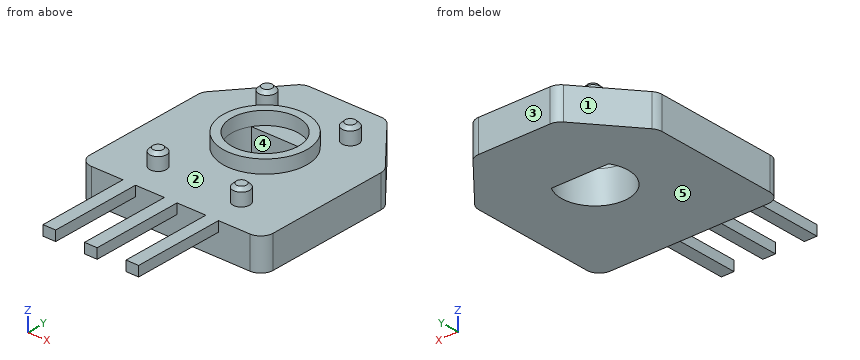
```python
from build123d import *
from build123d.topology import SkipClean

# Parameters (mm, degrees)
BOSS_EXTRUDE1_DEPTH = 1.93
SKETCH2_R           = 2.5
SKETCH2_R_2         = 2
BOSS_EXTRUDE2_DEPTH = 0.79
FILLET2_R           = 0.75
SKETCH5_R           = 0.5
BOSS_EXTRUDE4_DEPTH = 0.97
CHAMFER1_SIZE       = 0.2
SKETCH6_W           = 0.76
SKETCH6_H           = 0.6
BOSS_EXTRUDE5_DEPTH = 5.5


with BuildPart() as part:
    # Sketch1 → Boss-Extrude1 (new body)
    with BuildSketch(Plane.XY):
        Polygon((5.5, 0), (5.5, -6.5), (-5.5, -6.5), (-5.5, 0), (-5.5, 1.96), (-2.49602332, 5.54), (2.49602332, 5.54), (5.5, 1.96), align=None)
        with BuildLine():
            Line((-1.718566554, 1.023), (1.718566554, 1.023))
            ThreePointArc((1.718566554, 1.023), (0, -2), (-1.718566554, 1.023))
        make_face(mode=Mode.SUBTRACT)
    extrude(amount=BOSS_EXTRUDE1_DEPTH)

    # Sketch2 → Boss-Extrude2 (add)
    with SkipClean():  # the faces are left unmerged after this step: merging them gives an invalid solid
        with BuildSketch(Plane.XY.offset(1.93)):
            with Locations(Location((0, 0, 0), (0, 0, 180))):
                Circle(SKETCH2_R)
            with Locations(Location((0, 0, 0), (0, 0, 149.236204264))):
                Circle(SKETCH2_R_2, mode=Mode.SUBTRACT)
        extrude(amount=BOSS_EXTRUDE2_DEPTH)

    # Fillet2
    fillet2_edges = [part.edges().sort_by_distance(p)[0] for p in [
        (5.5, -6.5, 0.965),
        (-5.5, -6.5, 0.965),
        (-5.5, 1.96, 0.965),
        (-2.49602332, 5.54, 0.965),
        (2.49602332, 5.54, 0.965),
        (5.5, 1.96, 0.965),
    ]]
    fillet(fillet2_edges, radius=FILLET2_R)

    # Sketch5 → Boss-Extrude4 (add)
    with SkipClean():  # the faces are left unmerged after this step: merging them gives an invalid solid
        with BuildSketch(Plane.XY.offset(1.93)):
            with Locations(Location((-2.5, -4.5, 0), (0, 0, 180))):
                Circle(SKETCH5_R)
            with Locations(Location((2.5, -4.5, 0), (0, 0, 180))):
                Circle(SKETCH5_R)
            with Locations(Location((2.5, 3, 0), (0, 0, 180))):
                Circle(SKETCH5_R)
            with Locations(Location((-2.5, 3, 0), (0, 0, 180))):
                Circle(SKETCH5_R)
        extrude(amount=BOSS_EXTRUDE4_DEPTH)

    # Chamfer1
    chamfer1_edges = [part.edges().sort_by_distance(p)[0] for p in [
        (3, -4.5, 2.9),
        (-2, -4.5, 2.9),
        (3, 3, 2.9),
        (-2, 3, 2.9),
    ]]
    chamfer(chamfer1_edges, length=CHAMFER1_SIZE)

    # Sketch6 → Boss-Extrude5 (add)
    with SkipClean():  # the faces are left unmerged after this step: merging them gives an invalid solid
        with BuildSketch(Plane.XZ.offset(6.5)):
            with Locations((-2.49, 1.63)):
                Rectangle(SKETCH6_W, SKETCH6_H)
            with Locations((0, 1.63)):
                Rectangle(SKETCH6_W, SKETCH6_H)
            with Locations((2.49, 1.63)):
                Rectangle(SKETCH6_W, SKETCH6_H)
        extrude(amount=BOSS_EXTRUDE5_DEPTH)


solid = part.part
```
Geometry: final body of the model. Coordinates: model frame, mm. Face numbers are marked on the shaded views. A direction names the side the tool comes from. Coordinates: 2 decimals unless noted, no trailing zeros. Loops run counter-clockwise (first coordinate to the right, second up) from the corner with the lowest first, then second, coordinate; pieces in that order, holes last. Notation, with made-up numbers: M 73,-7.75 L 102,-7.75 A7 cw 102,0.25 Z; hole C -6,4.25 d5. An arc over 180 degrees is marked long. Put each result on its own line as item: value.
(1) Cut plane D-D on y = -7.25. Return the cut outline in (x, z).
Answer sheet:
outline: M -2.87,1.33 L -2.11,1.33 L -2.11,1.93 L -2.87,1.93 Z; M -0.38,1.33 L 0.38,1.33 L 0.38,1.93 L -0.38,1.93 Z; M 2.11,1.33 L 2.87,1.33 L 2.87,1.93 L 2.11,1.93 Z
(2) Draft query along Y for the marked faces 3, 4 and 5. Return one class per face: pulls with the +Y half, pulls with the -Y half, needs draft (parallel to the pull), parting line crosses it, or undercut.
Answer sheet:
face 3: pulls with the +Y half
face 4: undercut
face 5: needs draft
(3) Cut plane B-B on z = 2.2. Return the cut outline in (x, y), then the cut area to 3 significant figures.
Answer sheet:
outline: C -2.5,-4.5 d1; C -2.5,3 d1; C 0,0 d5; C 2.5,-4.5 d1; C 2.5,3 d1; hole C 0,0 d4
area: 10.2 mm^2
(4) First-contact query: pin 1 (2.5 mm diameter, centred on x = -1, y = 0, fed in from +Z); pin 2 (0.8 mm diameter, centred on x = 0, y = -9, fed in from -Z); pin 3 (3 mm diameter, centred on x = 0, y = 0, fed in from +Z). Flat tips, straight axial feed; report the tip coordinate or a pass-through.
Answer sheet:
pin 1: stops at z = 2.72
pin 2: stops at z = 1.33
pin 3: stops at z = 1.93
(5) Material intervals for probe 1 along X at (y, z) = (-7.75, 1.4); probe 2 along Y at (x, z) = (0, 2.65); probe 3 along X at (y, z) = (0, 1.05), sorted ascending.
Answer sheet:
probe 1: x = -2.87 to -2.11, -0.38 to 0.38, 2.11 to 2.87
probe 2: y = -2.5 to -2, 2 to 2.5
probe 3: x = -5.5 to -2, 2 to 5.5
(6) Cut plane C-C on x = 0. Return the cut outline in (y, z), then the cut area to 3 significant figures.
Answer sheet:
outline: M -12,1.33 L -6.5,1.33 L -6.5,0 L -2,0 L -2,2.72 L -2.5,2.72 L -2.5,1.93 L -12,1.93 Z; M 1.02,0 L 5.54,0 L 5.54,1.93 L 2.5,1.93 L 2.5,2.72 L 2,2.72 L 2,1.93 L 1.02,1.93 Z
area: 21.5 mm^2
(7) Access query for the marked faces 1 and 2. Directions: +Z, -Z, +X, -X, +Y, -Y. A direction counts if a zero-diameter tool reaches every point of the face in a straight line with its end or side. Return the directions, or none.
Answer sheet:
face 1: +Z, -Z, -X, +Y
face 2: +Z
(8) Cut plane A-A on y = 0. Return the cut outline in (x, z), then the cut area to 3 significant figures.
Answer sheet:
outline: M -5.5,0 L -2,0 L -2,2.72 L -2.5,2.72 L -2.5,1.93 L -5.5,1.93 Z; M 2,0 L 5.5,0 L 5.5,1.93 L 2.5,1.93 L 2.5,2.72 L 2,2.72 Z
area: 14.3 mm^2
